The listing builds one solid part. Answer for the finished solid, in the listing's coordinates (mm). Face numbers are marked on the shaded views. A direction names the side the tool comes from. Give positions to 0.01 mm unless a question says otherwise; leave off trailing zeros. Loops run counter-clockwise (first coordinate to the right, second up) from the corner with the lowest first, then second, coordinate; pieces in that order, holes last. Notation, with made-up numbers: M -31.5,35.5 L -5.5,35.5 A20 cw -5.5,47.5 Z; hole C -29.75,7.5 d10. An arc over 180 degrees is marked long. One line per item, written item: value. Start each with the question number.
Q1. Consider L1, parallel to Y at x = -44.5, z = -130.25; L2, parallel to X at y = 40, z = -139.75; L3, parallel to X at y = 21.5, z = -132.5. Determine where each line is inside the solid, lowest interval first.
Q2. A cutting plane is placed at C-C, the plane x = -5. Determine the outline of the cut face in (y, z).
Q3. A cutting plane is placed at D-D, the plane y = -6.5. Determine the outline of the cut face in (x, z), and give its area (3 significant figures).
Q4. Flat-ended cylindrical pins translate along their axes: pin 1 (12.5 mm diameter, centred on x = -36.5, z = -131, fed in from -Y); pin 2 (8 mm diameter, centred on y = -3.5, z = -138.5, fed in from +X); pin 3 (4 mm diameter, centred on x = -37.5, z = -140, fed in from +Y); pin 4 (8 mm diameter, centred on x = -10, y = 20, fed in from -Z). Find the tip coordinate at first contact, or state that the pin passes through.
Q5. For the marked faces 1 and 2, determine the directions among +Z, -Z, +X, -X, +Y, -Y from which every point of the face is accessible in a straight line to the end or side of a thin tool.
Q6. A cutting plane is placed at A-A, the plane y = 34.5. Determine the outline of the cut face in (x, z), and give its area (3 significant figures).
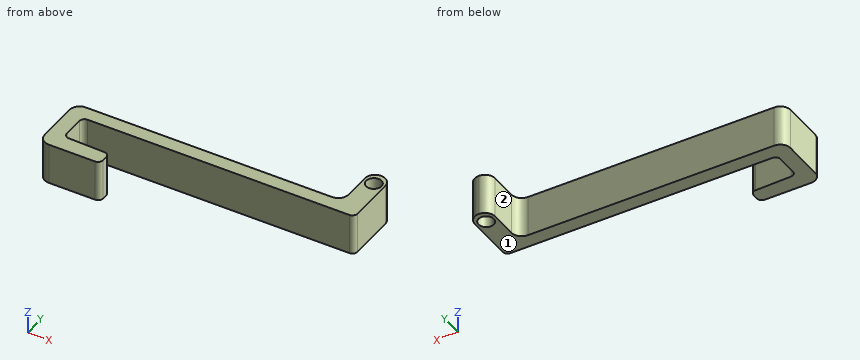
from build123d import *

# Parameters (mm, degrees)
F0_R     = 4.7625
F1_DEPTH = 25.4
F2_ANGLE = 90


with BuildPart() as f1:
    # F0 (on Right) → F1 (new body)
    with BuildSketch(Plane.YZ):
        with BuildLine():
            Line((-20.40446, 20.59559), (-17.143665, 20.59559))
            ThreePointArc((-17.143665, 20.59559), (-14.929557, 21.494991), (-13.969856, 23.683636))
            Line((-13.969856, 23.683636), (-13.356482, 46.071825))
            ThreePointArc((-13.356482, 46.071825), (-12.39678, 48.260471), (-10.182672, 49.159872))
            Line((-10.182672, 49.159872), (2.603122, 49.159872))
            ThreePointArc((2.603122, 49.159872), (4.848186, 48.229936), (5.778122, 45.984872))
            Line((5.778122, 45.984872), (5.778122, -115.927688))
            ThreePointArc((5.778122, -115.927688), (6.708058, -118.172752), (8.953122, -119.102688))
            Line((8.953122, -119.102688), (37.528122, -119.102688))
            ThreePointArc((37.528122, -119.102688), (42.01825, -117.242816), (43.878122, -112.752688))
            ThreePointArc((43.878122, -112.752688), (42.01825, -108.26256), (37.528122, -106.402688))
            Line((37.528122, -106.402688), (20.87054, -106.402688))
            ThreePointArc((20.87054, -106.402688), (16.380412, -104.542816), (14.52054, -100.052688))
            Line((14.52054, -100.052688), (14.52054, 52.34559))
            ThreePointArc((14.52054, 52.34559), (12.660668, 56.835718), (8.17054, 58.69559))
            Line((8.17054, 58.69559), (-17.22946, 58.69559))
            ThreePointArc((-17.22946, 58.69559), (-21.719588, 56.835718), (-23.57946, 52.34559))
            Line((-23.57946, 52.34559), (-23.57946, 23.77059))
            ThreePointArc((-23.57946, 23.77059), (-22.649524, 21.525526), (-20.40446, 20.59559))
        make_face()
        with Locations((36.073726, -112.88275)):
            Circle(F0_R, mode=Mode.SUBTRACT)
    extrude(amount=F1_DEPTH)


with BuildPart() as f1_1:
    # F2: moved
    add(f1.part.rotate(Axis((25.4, 23.240622, -119.102688), (0, -1, 0)), F2_ANGLE))


solid = f1_1.part
Answer block:
1. L1: 5.78 to 14.52
1. L2: 13.2 to 16.48, 21.88 to 24.9
1. L3: 12.7 to 25.4
2. outline: M 5.78,-144.5 L 14.52,-144.5 L 14.52,-119.1 L 5.78,-119.1 Z
3. outline: M -152.4,-144.5 L -142.86,-144.5 L -142.86,-119.1 L -152.4,-119.1 Z
3. area: 242 mm^2
4. pin 1: y = 5.78
4. pin 2: x = -142.86
4. pin 3: y = 14.52
4. pin 4: through
5. face 1: -Z, +X, -X, +Y, -Y
5. face 2: +Z, -Z, -X, +Y
6. outline: M 12.7,-144.5 L 14.69,-144.5 L 14.69,-119.1 L 12.7,-119.1 Z; M 23.68,-144.5 L 25.4,-144.5 L 25.4,-119.1 L 23.68,-119.1 Z
6. area: 94.2 mm^2
